Here's the drawing with two shaded views (mm, measured from the low corner). I have some questions. A direction names the side the tool comes from. Coordinates: 2 decimals unless noted, no trailing zeros. Write each loop counter-clockwise with the first axis right and the second up, starting at its lowest first coordinate (ties: lowest second). Pieces come first, ordered by that corner, then holes.
Item 1: I'm going to push flat-ended pins straight in: pin 1 Ø3.5 at (x, z) = (110, 80) entering from +Y; pin 2 Ø1.5 at (x, y) = (27.5, 95) entering from -Z; pin 3 Ø2.5 at (y, z) = (27.5, 79) entering from -X; pin 4 Ø10 at (x, z) = (39.5, 20.5) entering from +Y. Where does each tip first touch, or does it pass through?
Item 2: If I drill on line 1 (Z direction, x = 15.5, y = 110); line 2 (Z direction, x = 28.4, y = 110); line 3 (X direction, y = 101, z = 65.5), over which ranges is the centre line in solid material (lowest first)?
Item 3: For the marked faces 1, 2, 3, 4 and 5, which set-ups out of +Z, -Z, +X, -X, +Y, -Y let a thin tool reach every point of the face, with its end or its side?
Item 4: If we section it at D-D (x = 19): Please give me the cut outline in (y, z), then the cut area to 3 significant figures.
Item 5: If we section it at B-B (z = 27): Please give me the cut outline in (x, y).
Item 6: If we section it at C-C (y = 12): Please give me the cut outline in (x, z), then the cut area to 3 significant figures.
Item 7: If we section it at A-A (y = 110): Please give me the cut outline in (x, z), then the cut area to 3 significant figures.
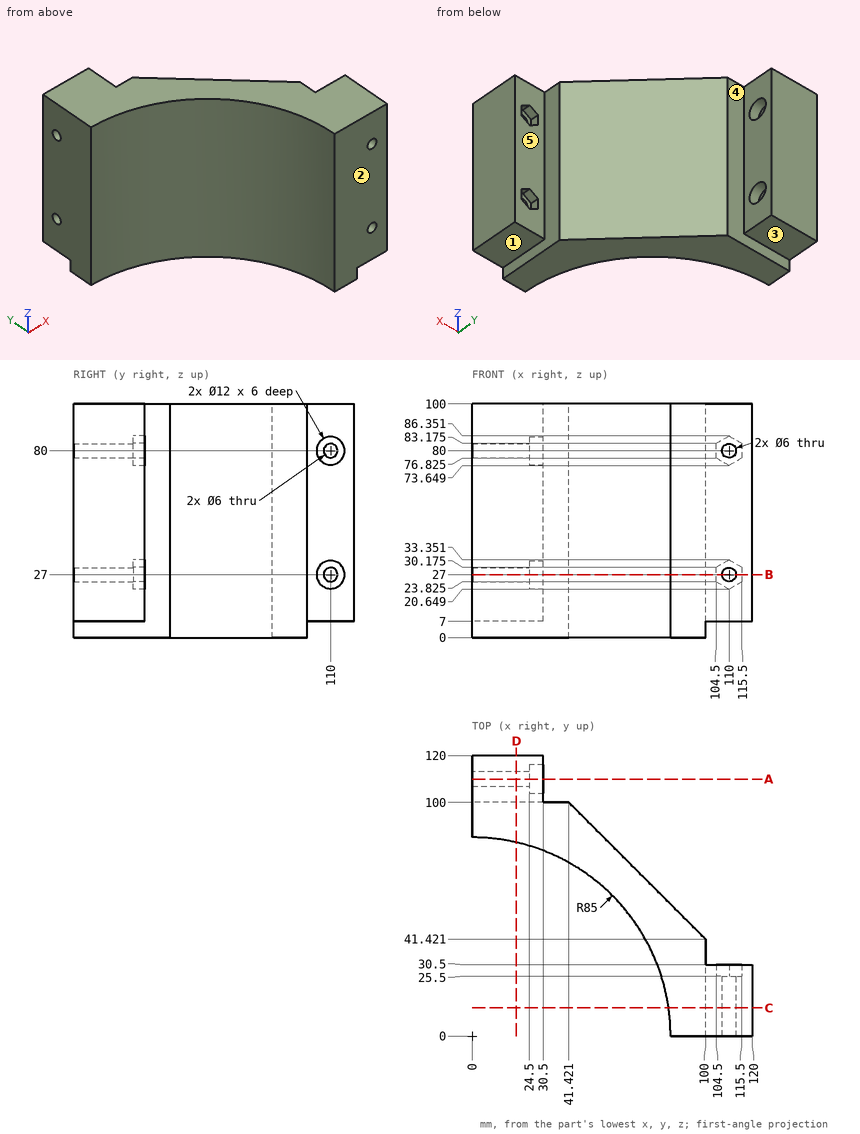
Answer list:
1. pin 1: passes through
1. pin 2: stops at z = 0
1. pin 3: stops at x = 79.99
1. pin 4: stops at y = 100
2. line 1: z = 7 to 24, 30 to 77, 83 to 100
2. line 2: z = 7 to 21, 33 to 74, 86 to 100
2. line 3: x = 0 to 30.5
3. face 1: -Z, +X, +Y, -Y
3. face 2: +Z, -Z, +X, -X, -Y
3. face 3: -Z, +X, -X, +Y
3. face 4: -Z, +X, +Y
3. face 5: +Z, -Z, +X, +Y
4. outline: (82.85, 0) - (100, 0) - (100, 7) - (120, 7) - (120, 100) - (82.85, 100) - close; hole circle Ø6 at (110, 27); hole circle Ø6 at (110, 80)
4. area: 3,520 mm2
5. outline: (0, 85) arc R85 cw to (85, 0) - (107, 0) - (107, 25.5) - (104.5, 25.5) - (104.5, 30.5) - (100, 30.5) - (100, 41.42) - (41.42, 100) - (30.5, 100) - (30.5, 104) - (24.5, 104) - (24.5, 107) - (0, 107) - close; (0, 113) - (24.5, 113) - (24.5, 116) - (30.5, 116) - (30.5, 120) - (0, 120) - close; (113, 0) - (120, 0) - (120, 30.5) - (115.5, 30.5) - (115.5, 25.5) - (113, 25.5) - close
6. outline: (84.15, 0) - (100, 0) - (100, 7) - (120, 7) - (120, 100) - (84.15, 100) - close; hole circle Ø6 at (110, 27); hole circle Ø6 at (110, 80)
6. area: 3,390 mm2
7. outline: (0, 7) - (30.5, 7) - (30.5, 21) - (24.5, 21) - (24.5, 24) - (0, 24) - close; (0, 30) - (24.5, 30) - (24.5, 33) - (30.5, 33) - (30.5, 74) - (24.5, 74) - (24.5, 77) - (0, 77) - close; (0, 83) - (24.5, 83) - (24.5, 86) - (30.5, 86) - (30.5, 100) - (0, 100) - close
7. area: 2,400 mm2
